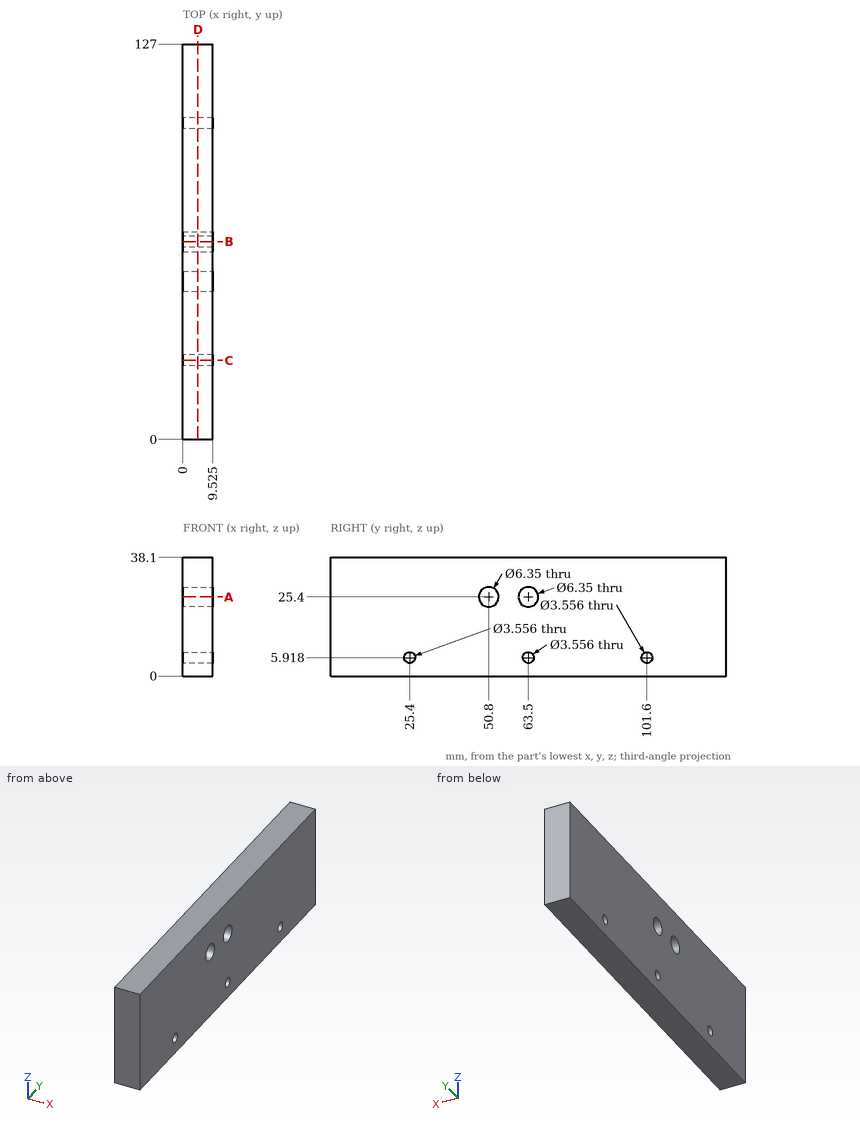
Can you work these out from the drawing? Everything is in mm from the part's minimum corner. Give positions to 0.01 mm unless a question says otherwise; leave off trailing zeros. Loops run counter-clockwise (first coordinate to the right, second up) from the corner with the lowest first, then second, coordinate; pieces in that order, holes last. Notation, with made-up numbers: (12.5, 41) -> (43.5, 41) arc R31 cw to (43.5, 70) -> close; hole circle Ø3 at (65, 37.5). An arc over 180 degrees is marked (long way). Write item = value, one per line.
1) Suppose I cut it at D-D on x = 4.75. Give the number of separate pieces and of enclosed holes in the cut face, then the cut area to 3 significant figures.
Check result:
separate_pieces = 1
enclosed_holes = 5
area = 4,750 mm2
2) Suppose I cut it at A-A on z = 25.4. Write out the boundary of the cut face in (x, y) (3 decimals).
Check result:
outline = (0, 0) -> (9.525, 0) -> (9.525, 47.625) -> (0, 47.625) -> close; (0, 53.975) -> (9.525, 53.975) -> (9.525, 60.325) -> (0, 60.325) -> close; (0, 66.675) -> (9.525, 66.675) -> (9.525, 127) -> (0, 127) -> close
3) Will this pin go through, and if not, where does the flat tip stop? pin 1 (3 mm diameter, centred on y = 25.4, z = 5.92, fed in from -X).
Check result:
pin_1 = through
4) I need wall thicknesses on L1, parallel to Y at x = 7.5, z = 25.4 (3 decimals); L2, parallel to Y at x = 9, z = 22.5; L3, parallel to Z at x = 4.75, y = 61. Which ranges of each line are inside material? Lowest first, please. Write a range as from..to.
Check result:
L1 = 0..47.625, 53.975..60.325, 66.675..127
L2 = 0..49.51, 52.09..62.21, 64.79..127
L3 = 0..23.44, 27.36..38.1
5) Suppose I cut it at B-B on y = 63.5. Write out the boundary of the cut face in (x, z) (1 decimal).
Check result:
outline = (0, 0) -> (9.5, 0) -> (9.5, 4.1) -> (0, 4.1) -> close; (0, 7.7) -> (9.5, 7.7) -> (9.5, 22.2) -> (0, 22.2) -> close; (0, 28.6) -> (9.5, 28.6) -> (9.5, 38.1) -> (0, 38.1) -> close
6) Suppose I cut it at C-C on y = 25.4. Write out the boundary of the cut face in (x, z) (1 decimal).
Check result:
outline = (0, 0) -> (9.5, 0) -> (9.5, 4.1) -> (0, 4.1) -> close; (0, 7.7) -> (9.5, 7.7) -> (9.5, 38.1) -> (0, 38.1) -> close
